Check sheet for the drawn part. Datum: minimum x, y, z corner. Units: mm. A direction names the side the tool comes from. Coordinates: 2 decimals unless noted, no trailing zeros. Order: outer loops, then holes, each group sorted by start corner. A loop starts at its lowest first (then second) coordinate and runs counter-clockwise, first axis right, second up. Notation, with made-up numbers: (57, -11) - (68, -11) arc R21 cw to (68, -3) - close; hole circle Ø11 at (-16.75, -25.75). An arc over 180 degrees is marked (long way). Answer as CSV lines item,"result". Start each with the question number.
1. Section check A-A (x = 180). Record the cut outline in (y, z).
2. Section check B-B (z = 30). Record the cut outline in (x, y).
3. Go/stop test with flat-tipped pins: pin 1 (3 mm diameter, centred on x = 46, z = 41.5, fed in from -Y); pin 2 (2 mm diameter, centred on y = 104, z = 27, fed in from +X); pin 3 (4 mm diameter, centred on y = 15.5, z = 12.5, fed in from -X). Record where each tip stops, or that it passes through.
4. Material ranges on L1, parallel to X at y = 1.3, z = 30; L2, parallel to Y at x = 29.5, z = 18.5; L3, parallel to X at y = 119, z = 7.5, recorded low to high. Write a range as [from, to].
5. Mould release check, pull along Y, two halves, no side actions. Record for the marked faces 1, 2 and 3: pulls with the +Y half, pulls with the -Y half, needs draft (parallel to the pull), parting line crosses it, or undercut.
6. Set-up check for the marked faces 4, 5 and 6: record each of +Z, -Z, +X, -X, +Y, -Y from which the full face is reachable in a straight line by a thin tool's end or side.
7. Section check D-D (y = 24). Record the cut outline in (x, z), and give its area (3 significant figures).
8. Section check C-C (z = 50.5). Record the cut outline in (x, y).
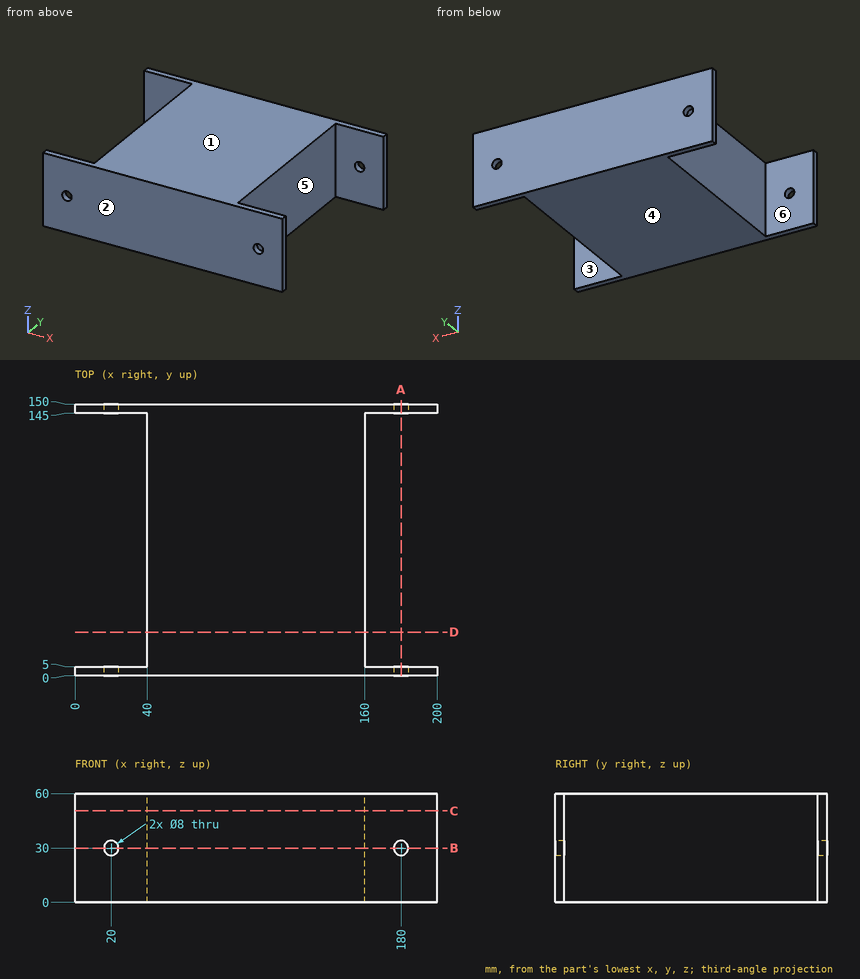
Evaluation:
1,outline,"(0, 0) - (5, 0) - (5, 26) - (0, 26) - close; (0, 34) - (5, 34) - (5, 60) - (0, 60) - close; (145, 0) - (150, 0) - (150, 26) - (145, 26) - close; (145, 34) - (150, 34) - (150, 60) - (145, 60) - close"
2,outline,"(0, 0) - (16, 0) - (16, 5) - (0, 5) - close; (0, 145) - (16, 145) - (16, 150) - (0, 150) - close; (24, 0) - (176, 0) - (176, 5) - (160, 5) - (160, 145) - (176, 145) - (176, 150) - (24, 150) - (24, 145) - (40, 145) - (40, 5) - (24, 5) - close; (184, 0) - (200, 0) - (200, 5) - (184, 5) - close; (184, 145) - (200, 145) - (200, 150) - (184, 150) - close"
3,pin 1,"stops at y = 0"
3,pin 2,"stops at x = 160"
3,pin 3,"stops at x = 40"
4,L1,"x = [0, 16], [24, 176], [184, 200]"
4,L2,"y = [0, 5], [145, 150]"
4,L3,"x = [40, 160]"
5,face 1,"needs draft"
5,face 2,"pulls with the -Y half"
5,face 3,"undercut"
6,face 4,"-Z, +X, -X, +Y, -Y"
6,face 5,"+Z, -Z, +X"
6,face 6,"+Z, -Z, -X"
7,outline,"(40, 0) - (160, 0) - (160, 60) - (40, 60) - close"
7,area,"7,200 mm²"
8,outline,"(0, 0) - (200, 0) - (200, 5) - (160, 5) - (160, 145) - (200, 145) - (200, 150) - (0, 150) - (0, 145) - (40, 145) - (40, 5) - (0, 5) - close"
